Print and shaded views of the part. All mm, measured from the part's lowest x, y and z. A direction names the side the tool comes from. Coordinates: 2 decimals unless noted, no trailing zeros. Order: outer loops, then holes, each group sorted by start corner. A loop starts at its lowest first (then second) coordinate and runs counter-clockwise, first axis right, second up. Notation, with made-up numbers: M 81,31.5 L 106,31.5 A12 cw 106,53.5 Z; hole C 69,-36 d9. An arc over 180 degrees is marked long. Use a Markdown table: item, result. Add a question column.
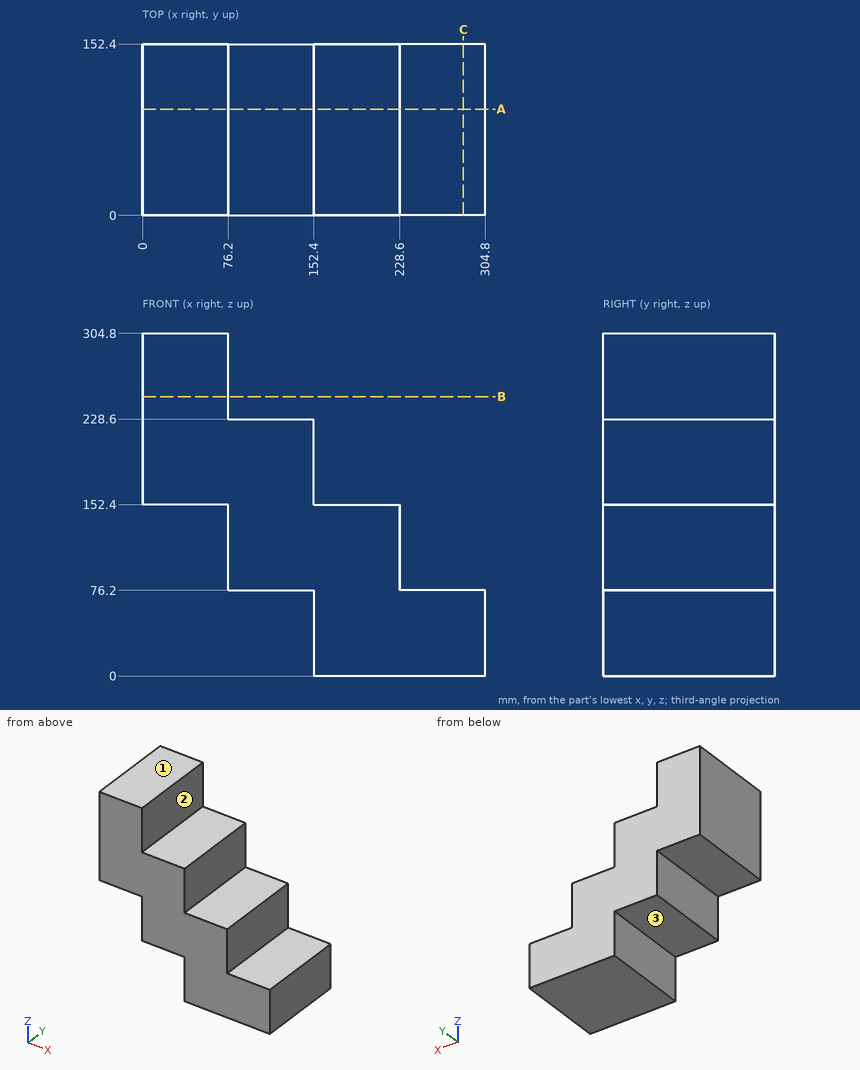
(1) Slice it at C-C on x = 285.5. Give the cut face in (y, z), and give its area (3 significant figures).
(2) Drop flat-ended pins along their axis: P1, Ø1, axis at x = 125, y = 49.5, coming from the -Z side; P2, Ø23, axis at x = 258.5, y = 63.5, coming from the +Z side; P3, Ø6, axis at y = 68.5, z = 52, coming from the -X side; P4, Ø1, axis at x = 220, y = 40, coming from the -Z side. Give the stop position or say it passes through.
(3) Which spindle directions (+Z, -Z, +X, -X, +Y, -Y) get a long thin tool onto all of the face, cutting with end or side? Do the marked faces 1, 2 and 3. Say none if no direction does.
(4) Slice it at A-A on y = 94.5. Give the cut face in (x, z).
(5) Drill centre lines: line 1 along X through (y, z) = (122.5, 208); line 2 along Z through (x, y) = (39, 27.5); line 3 along X through (y, z) = (59, 229.5). Where is each one in solid material? Low to high. Write a range as from..to.
(6) Slice it at B-B on z = 248.5. Give the cut face in (x, y).
Solutions:
| question | item | result |
|---|---|---|
| 1 | outline | M 0,0 L 152.4,0 L 152.4,76.2 L 0,76.2 Z |
| 1 | area | 11,600 mm² |
| 2 | P1 | z = 76.2 |
| 2 | P2 | z = 76.2 |
| 2 | P3 | x = 152.4 |
| 2 | P4 | z = 0 |
| 3 | face 1 | +Z, +X, -X, +Y, -Y |
| 3 | face 2 | +Z, +X, +Y, -Y |
| 3 | face 3 | -Z, -X, +Y, -Y |
| 4 | outline | M 0,152.4 L 76.2,152.4 L 76.2,76.2 L 152.4,76.2 L 152.4,0 L 304.8,0 L 304.8,76.2 L 228.6,76.2 L 228.6,152.4 L 152.4,152.4 L 152.4,228.6 L 76.2,228.6 L 76.2,304.8 L 0,304.8 Z |
| 5 | line 1 | 0..152.4 |
| 5 | line 2 | 152.4..304.8 |
| 5 | line 3 | 0..76.2 |
| 6 | outline | M 0,0 L 76.2,0 L 76.2,152.4 L 0,152.4 Z |
